Work out the finished part from the listing and answer in its coordinate system (mm). A direction names the side the tool comes from. Round coordinates to 2 decimals unless told otherwise and drop trailing zeros. Write each loop counter-clockwise with the first axis right and the second up, starting at its lowest first coordinate (ties: lowest second). Pieces come first, ordered by that corner, then holes. Notation, with made-up numbers: (-4, 81.25) -> (20, 81.25) arc R27 ccw to (20, 111.25) -> close; hole circle Ø8 at (43.25, -10). An arc over 180 degrees is marked (long way). Answer as a JSON object with one key per item and string values. Group by question number.
from build123d import *

# Parameters (mm, degrees)
F0_W     = 90
F0_H     = 120
F1_DEPTH = 30
F2_T     = -2.5
F3_R     = 1.25
F4_DEPTH = 25


with BuildPart() as f1:
    # F0 (on Front) → F1 (new body)
    with BuildSketch(Plane.XZ):
        with Locations((-45, 60)):
            Rectangle(F0_W, F0_H)
    extrude(amount=F1_DEPTH)

    # F2
    f2_openings = [f1.faces().sort_by_distance(p)[0] for p in [
        (-45, -30, 60),
    ]]
    offset(amount=F2_T, openings=f2_openings)

    # F3 (on face) → F4 (cut)
    with BuildSketch(Plane(origin=(0, 0, 0), x_dir=(1, 0, 0), z_dir=(0, 0, -1))):
        with Locations((-45, 15)):
            Circle(F3_R)
    extrude(amount=-F4_DEPTH, mode=Mode.SUBTRACT)


solid = f1.part
1) A cutting plane is placed at D-D on x = -18. Determine the outline of the cut face in (y, z).
2) A cutting plane is placed at B-B on x = -45. Determine the outline of the cut face in (y, z).
3) A cutting plane is placed at C-C on y = -15. Determine the outline of the cut face in (x, z).
4) Each of these flat-tipped pins is pushed along its axis until it touches: P1, Ø3, axis at x = -21.5, z = 43.5, coming from the -Y side; P2, Ø1.5, axis at x = -45, y = -15, coming from the -Z side. Where does it stop, or does it pass through?
5) A tool of negligible diameter and unlimited length cuts with its end or side. For faces 1 (the face through (-45.921, -15.845, 1.232)), 2 (the face through (0, -15, 59)), 3 (the face through (-2.5, -16, 59)), from which of +Z, -Z, +X, -X, +Y, -Y can it reach the whole face along a straight path? Write none if from no direction.
6) Straight lines are drawn through the part: L1, parallel to Z at x = -59, y = -8.5; L2, parallel to Y at x = -45, z = 1.35; L3, parallel to X at y = -15, z = 0.8. For each, find the intervals that lie inside material, in ascending order.
7) For a pull along X with two mould halves and no side action, classify faces 4 (the face through (-46, 0, 61)), 5 (the face through (-46, -2.5, 61)), 6 (the face through (-90, -15, 59)) as released by +X, released by -X, zero draft, split by the parting line, or undercut.
8) A cutting plane is placed at A-A on z = 98. Determine the outline of the cut face in (x, y), plus the area to 4 significant figures.
Established:
{
 "1": {"outline": "(-30, 0) -> (0, 0) -> (0, 120) -> (-30, 120) -> (-30, 117.5) -> (-2.5, 117.5) -> (-2.5, 2.5) -> (-30, 2.5) -> close"},
 "2": {"outline": "(-30, 0) -> (-16.25, 0) -> (-16.25, 2.5) -> (-30, 2.5) -> close; (-30, 117.5) -> (-2.5, 117.5) -> (-2.5, 2.5) -> (-13.75, 2.5) -> (-13.75, 0) -> (0, 0) -> (0, 120) -> (-30, 120) -> close"},
 "3": {"outline": "(-90, 0) -> (-46.25, 0) -> (-46.25, 2.5) -> (-87.5, 2.5) -> (-87.5, 117.5) -> (-2.5, 117.5) -> (-2.5, 2.5) -> (-43.75, 2.5) -> (-43.75, 0) -> (0, 0) -> (0, 120) -> (-90, 120) -> close"},
 "4": {"P1": "stops at y = -2.5", "P2": "stops at z = 117.5"},
 "5": {"face 1": "-Z", "face 2": "+Z, -Z, +X, +Y, -Y", "face 3": "-Y"},
 "6": {"L1": "z = 0 to 2.5, 117.5 to 120", "L2": "y = -30 to -16.25, -13.75 to 0", "L3": "x = -90 to -46.25, -43.75 to 0"},
 "7": {"face 4": "zero draft", "face 5": "undercut", "face 6": "released by -X"},
 "8": {"outline": "(-90, -30) -> (-87.5, -30) -> (-87.5, -2.5) -> (-2.5, -2.5) -> (-2.5, -30) -> (0, -30) -> (0, 0) -> (-90, 0) -> close", "area": "362.5 mm²"}
}
